Autodesk Inventor part; units mm, degrees
ref_plane "YZ Plane" through (0, 0, 0) normal (1, 0, 0) x (0, 1, 0)
ref_plane "XZ Plane" through (0, 0, 0) normal (0, 1, 0) x (-1, 0, 0)
ref_plane "Work Plane1" through (0, 0, -50.8) normal (0, 0, 1) x (1, 0, 0)
sketch "Sketch1" plane through (0, 0, -50.8) normal (0, 0, 1) x (1, 0, 0)
  line L0 (-11.933319, 0) -> (16.362179, 0)
  point P0 (0, 0)
ref_plane "Work Plane2" through (-11.933319, 0, -50.8) normal (0, -0.0871557, 0.9961947) x (1, 0, 0)
sketch "Sketch2" plane through (-11.933319, 0, -50.8) normal (0, -0.0871557, 0.9961947) x (1, 0, 0)
  line L0 (20.901803, 66.92299) -> (20.901803, 43.564038)
  line L1 (18.251803, 42.008516) -> (18.251803, 68.335864)
  line L2 (18.251803, 42.008516) -> (20.901803, 42.008516)
  line L3 (-146.748197, 17.044024) -> (-146.748197, 40.704766)
  line L4 (-149.398197, 17.044024) -> (-149.398197, 40.704766)
  line L5 (-149.398197, 42.001169) -> (-149.398197, 42.510921)
  line L6 (-146.748197, 17.044024) -> (-149.398197, 17.044024)
  arc A0 (-146.748197, 17.044024) -> (18.251803, 42.008516) centre (-77.743959, 118.72499) ccw
  arc A1 (-149.398197, 17.044024) -> (20.901803, 42.008516) centre (-75.863874, 108.764811) ccw
  line L7 (-121.884258, 0.588457) -> (-124.244108, -1.791919)
  arc A2 (-154.040418, 23.398782) -> (-124.244108, -1.791919) centre (-114.93586, 39.435485) ccw
  line L8 (-154.040418, 23.398782) -> (-144.892983, 23.398782)
  line L9 (-144.892983, 23.398782) -> (-144.394088, 15.485637)
  line L10 (-21.699981, 4.427512) -> (-19.714804, 2.459452)
  arc A3 (-19.714804, 2.459452) -> (22.454201, 45.29191) centre (-43.243229, 67.797577) ccw
  line L11 (22.454201, 45.29191) -> (15.711222, 45.29191)
  line L12 (15.711222, 45.29191) -> (15.711222, 38.933181)
  point P0 (11.933319, 4.427512)
extrude "Extrusion1" add sketch "Sketch2" along normal mid plane 25.4
fillet "Fillet1" radius 12.7 4 edges at (-32.6407, 2.3235, -37.8482) (-32.6407, 4.5373, -63.1516) (-134.9975, -1.7063, -38.2008) (-134.9975, 0.5074, -63.5041)
properties part number "thigh_strap_02"
Build history of the part. All positions in model axes, mm. A direction names the side the tool comes from. Coordinates: 2 decimals unless noted, no trailing zeros. Write each loop counter-clockwise with the first axis right and the second up, starting at its lowest first coordinate (ties: lowest second). Pieces come first, ordered by that corner, then holes. Notation, with made-up numbers: (83.25, -27.75) -> (107.25, -27.75) arc R25 cw to (107.25, 8.25) -> close; hole circle Ø1 at (-39.75, 58.5). An arc over 180 degrees is marked (long way). Use CSV: the item, a comma, the result in double quotes. Start each with the question number.
Q1. Cut at B-B, the plane x = -77. List the corners of the cut face in (y, z), then the cut area to 3 significant figures.
Q2. Drill centre lines: probe 1 along X at (y, z) = (6.5, -60.5); probe 2 along X at (y, z) = (20.5, -38); probe 3 along X at (y, z) = (23, -57.5). Where is each one in solid material? Low to high.
Q3. Flat gauge pins, fed straight in: pin 1 Ø4 at (y, z) = (34.5, -43) entering from -X; pin 2 Ø5 at (y, z) = (40.5, -54.5) entering from -X; pin 3 Ø2.5 at (y, z) = (42.5, -43.5) entering from -X. Where does each tip first touch, or does it go through?
Q4. Pull direction X, two halves, no side cores. Call faces 1 (the cylindrical face through (-153.939, 6.966, -50.369)), 2 (the cylindrical face through (-28.869, 4.271, -41.313)), 3 (the cylindrical face through (-29.008, 5.697, -59.217)), 4 (the flat face through (-71.6, -2.54, -63.77)): released by +X, released by -X, zero draft, split by the parting line, or undercut.
Q5. 3-axis set-ups, long thin cutter, end or side, ignore diameter. For faces 5 (the flat face through (3.778, 42, -47)), 6 (the cylindrical face through (-5.385, 19.33, -49.287)), 7 (the cylindrical face through (-138.94, 1.63, -59.77)): which of +Z, -Z, +X, -X, +Y, -Y reach the whole face in a straight line?
Q6. Cut at A-A, the plane x = -55. List the corners of the cut face in (y, z).
Checked values:
1,outline,"(-9.37, -38.87) -> (-7.16, -64.17) -> (-2.38, -63.76) -> (-4.6, -38.45) -> close"
1,area,"122 mm²"
2,probe 1,"x = -152.24 to -137.74, -41.61 to -31.38, -27.5 to -24.23"
2,probe 2,"x = -165.16 to -156.71, -14.48 to -3.38"
2,probe 3,"x = -165.52 to -156.76, -13.46 to -2.69"
3,pin 1,"stops at x = -1.59"
3,pin 2,"stops at x = 2.56"
3,pin 3,"stops at x = 3.78"
4,face 1,"released by -X"
4,face 2,"undercut"
4,face 3,"undercut"
4,face 4,"zero draft"
5,face 5,"+Z, -X, +Y"
5,face 6,"-Z, +X, -Y"
5,face 7,"-Z"
6,outline,"(-5.22, -38.51) -> (-3, -63.81) -> (1.94, -63.38) -> (-0.28, -38.08) -> close"
